Read the model definition and answer for the solid it produces. Units are mm, in the model's axes. Face numbers are marked on the shaded views. A direction names the side the tool comes from. Round coordinates to 2 decimals unless told otherwise and drop trailing zeros. Write each loop counter-clockwise with the first axis right and the second up, starting at its lowest first coordinate (ties: lowest second). Pieces come first, ordered by that corner, then holes. Notation, with made-up numbers: (-5.5, 57.5) -> (34.5, 57.5) arc R18 ccw to (34.5, 69.5) -> close; hole circle Ø6 at (0.5, 15.5). An arc over 180 degrees is marked (long way). Return JSON: item names as keys, results as strings. Group by question number.
(1) A cutting plane is placed at A-A on y = 0. Give the vertices of the cut face in (x, z), then the cut area to 3 significant figures.
(2) Straight lines are drawn through the part: line 1 (Y direction, x = 35, z = -1); line 2 (Y direction, x = 13, z = -26.5); line 3 (Y direction, x = -40.5, z = 0). For each, find the intervals that lie inside material, in ascending order.
(3) A cutting plane is placed at D-D on z = 0. Give the vertices of the cut face in (x, y), then the cut area to 3 significant figures.
(4) For the marked faces 4, 5 and 6, determine the directions among +Z, -Z, +X, -X, +Y, -Y from which every point of the face is accessible in a straight line to the end or side of a thin tool.
(5) A cutting plane is placed at B-B on x = -35.56. Give the vertices of the cut face in (y, z), then the cut area to 3 significant figures.
(6) A cutting plane is placed at C-C on x = 0. Give the vertices of the cut face in (y, z).
(7) Given pin 1 (12 mm diameter, centred on x = -35.56, y = 0, fed in from +Z); pin 2 (3 mm diameter, centred on x = -37.5, z = -20, fed in from +Y); pin 3 (2 mm diameter, centred on x = 39, z = 23, fed in from -Y), each flat-ended and moving along its own axis, determine where each tip first touches the part or whether it passes through.
(8) The mould has two halves that part along X. Classify the marked faces 1, 2 and 3: released by +X, released by -X, zero draft, split by the parting line, or undercut.
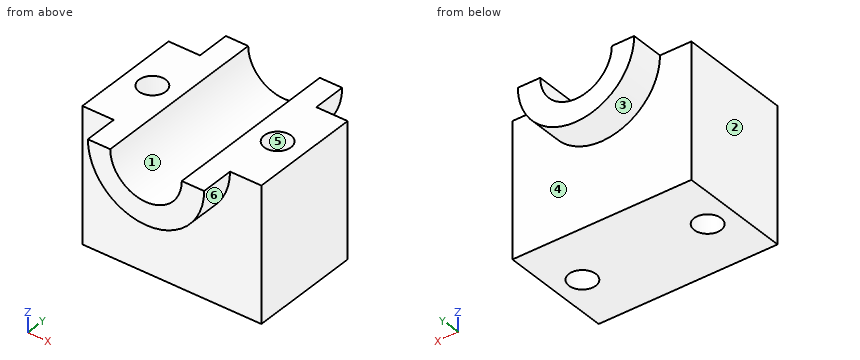
```python
from build123d import *

# Parameters (mm, degrees)
F0_W     = 101.6
F0_H     = 76.2
F1_DEPTH = 31.75
F3_DEPTH = 50.8
F5_DEPTH = 76.2
F6_R     = 7.62
F7_DEPTH = 76.2


with BuildPart() as f1:
    # F0 (on Front) → F1 (new body, symmetric)
    with BuildSketch(Plane.XZ):
        Rectangle(F0_W, F0_H)
    extrude(amount=F1_DEPTH, both=True)

    # F2 (on Front) → F3 (join, symmetric)
    with BuildSketch(Plane.XZ):
        with BuildLine():
            ThreePointArc((20.32, 38.1), (0, 17.78), (-20.32, 38.1))
            Line((-20.32, 38.1), (-33.02, 38.1))
            ThreePointArc((-33.02, 38.1), (0, 5.08), (33.02, 38.1))
            Line((33.02, 38.1), (20.32, 38.1))
        make_face()
    extrude(amount=F3_DEPTH, both=True)

    # F4 (on face) → F5 (cut)
    with BuildSketch(Plane.XZ.offset(31.75)):
        with BuildLine():
            Line((20.32, 38.1), (-20.32, 38.1))
            ThreePointArc((-20.32, 38.1), (0, 17.78), (20.32, 38.1))
        make_face()
    extrude(amount=-F5_DEPTH, mode=Mode.SUBTRACT)

    # F6 (on face) → F7 (cut)
    with BuildSketch(Plane.XY.offset(38.1)):
        with Locations((-35.56, 0)):
            Circle(F6_R)
        with Locations((35.56, 0)):
            Circle(F6_R)
    extrude(amount=-F7_DEPTH, mode=Mode.SUBTRACT)


solid = f1.part
```
Checks:
{
 "1": {"outline": "(-50.8, -38.1) -> (-43.18, -38.1) -> (-43.18, 38.1) -> (-50.8, 38.1) -> close; (-27.94, -38.1) -> (27.94, -38.1) -> (27.94, 38.1) -> (20.32, 38.1) arc R20.32 cw to (-20.32, 38.1) -> (-27.94, 38.1) -> close; (43.18, -38.1) -> (50.8, -38.1) -> (50.8, 38.1) -> (43.18, 38.1) -> close", "area": "4,770 mm^2"},
 "2": {"line 1": "y = -31.75 to -7.6, 7.6 to 31.75", "line 2": "y = -31.75 to 31.75", "line 3": "y = -31.75 to -5.8, 5.8 to 31.75"},
 "3": {"outline": "(-50.8, -31.75) -> (50.8, -31.75) -> (50.8, 31.75) -> (-50.8, 31.75) -> close; hole circle Ø15.24 at (-35.56, 0); hole circle Ø15.24 at (35.56, 0)", "area": "6,090 mm^2"},
 "4": {"face 4": "-Z, +Y", "face 5": "+Z, -Z", "face 6": "-Z, -Y"},
 "5": {"outline": "(-31.75, -38.1) -> (-7.62, -38.1) -> (-7.62, 38.1) -> (-31.75, 38.1) -> close; (7.62, -38.1) -> (31.75, -38.1) -> (31.75, 38.1) -> (7.62, 38.1) -> close", "area": "3,680 mm^2"},
 "6": {"outline": "(-50.8, 5.08) -> (-31.75, 5.08) -> (-31.75, -38.1) -> (31.75, -38.1) -> (31.75, 5.08) -> (50.8, 5.08) -> (50.8, 17.78) -> (-50.8, 17.78) -> close"},
 "7": {"pin 1": "passes through", "pin 2": "stops at y = 31.75", "pin 3": "stops at y = -31.75"},
 "8": {"face 1": "undercut", "face 2": "released by -X", "face 3": "split by the parting line"}
}
